The listing builds one solid part. Answer for the finished solid, in the listing's coordinates (mm). Face numbers are marked on the shaded views. A direction names the side the tool comes from. Round coordinates to 2 decimals unless told otherwise and drop trailing zeros. Write each loop counter-clockwise with the first axis right and the second up, starting at its lowest first coordinate (ties: lowest second). Pieces come first, ordered by that corner, then holes. Notation, with made-up numbers: (68, 7) - (126, 7) arc R32 cw to (126, 38) - close; hole circle Ø2 at (49, 79.5). An arc over 180 degrees is marked (long way). Return JSON: item names as keys, results as strings. Group by question number.
(1) Section B-B, the plane x = 28.5 is taken. Give the number of separate pieces and of enclosed holes in the cut face, then the cut area to 3 significant figures.
(2) Each of these flat-tipped pins is pushed along its axis until it touches: pin 1 (20 mm diameter, centred on y = -25.5, z = 6.5, fed in from +X); pin 2 (6 mm diameter, centred on x = -30.5, y = -12.5, fed in from +Z); pin 3 (3 mm diameter, centred on x = 7.5, y = -31.5, fed in from -Z). Where does it stop, or does it pass through?
(3) Determine the mould class of the marked faces 1, 2 and 3 for opening direction Z: +Z half, -Z half, draft (parallel to the pull), parting line (faces both ways), or undercut.
(4) Section A-A, the plane z = 0 is taken. Write down the section's boundary in (x, y), then the cut area to 3 significant figures.
(5) Which of the six approach directions +Z, -Z, +X, -X, +Y, -Y give full straight-line access (tool end or side, diameter ignored) to the marked faces 4, 5, 6 and 7?
(6) Find the intervals of material crossed by line 1 along Z through (x, y) = (0, -18) (3 decimals); line 2 along X through (y, z) = (-28.5, -25.5); line 3 along Z through (x, y) = (-0.5, -4), in increasing order. Write a range as [from, to].
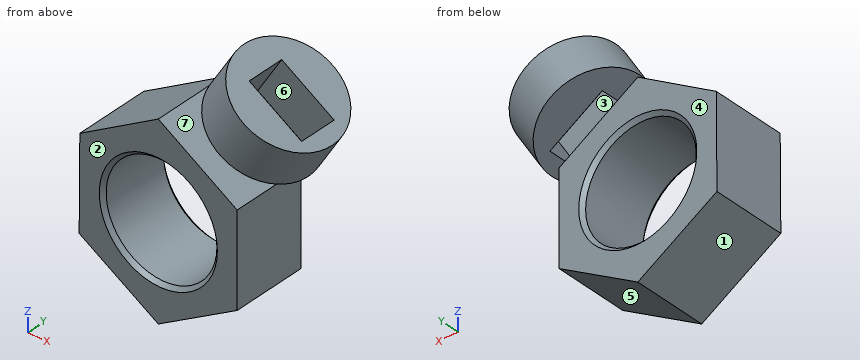
```python
from build123d import *

# Parameters (mm, degrees)
F0_R     = 30
F1_DEPTH = 40
F2_SIZE  = 2
F3_R     = 27.9010613337
F3_W     = 33.2406070083
F3_H     = 20.383390598
F4_DEPTH = 25


with BuildPart() as f1:
    # F0 (on Front) → F1 (new body)
    with BuildSketch(Plane.XZ):
        Polygon((0, 51.3005799085), (-42.5238697261, 25), (-42.8737902332, -24.9987755414), (0, -50.724990013), (42.7005271465, -24.7122050523), (42.7005271465, 25.2877949477), align=None)
        Circle(F0_R, mode=Mode.SUBTRACT)
    extrude(amount=F1_DEPTH)

    # F2
    f2_edges = [f1.edges().sort_by_distance(p)[0] for p in [
        (-30, -40, 0),
        (-30, 0, 0),
    ]]
    chamfer(f2_edges, length=F2_SIZE)

    # F3 (on face) → F4 (join)
    with BuildSketch(Plane(origin=(22.7930452708, 0, 37.4152575284), x_dir=(0.8540105429, 0, -0.5202556992), z_dir=(0.5202556992, 0, 0.8540105429))):
        Circle(F3_R)
        with Locations((2.8576394543, -0.7141805254)):
            Rectangle(F3_W, F3_H, mode=Mode.SUBTRACT)
    extrude(amount=F4_DEPTH)


solid = f1.part
```
Working result:
{
 "1": {"separate pieces": "3", "enclosed holes": "0", "area": "2,940 mm^2"},
 "2": {"pin 1": "stops at x = 42.7", "pin 2": "stops at z = 34.29", "pin 3": "stops at z = -47.07"},
 "3": {"face 1": "-Z half", "face 2": "draft", "face 3": "undercut"},
 "4": {"outline": "(-42.7, -40) - (-32, -40) - (-30, -38) - (-30, -2) - (-32, 0) - (-42.7, 0) - close; (30, -38) - (32, -40) - (42.7, -40) - (42.7, 0) - (32, 0) - (30, -2) - close", "area": "1,010 mm^2"},
 "5": {"face 4": "-Z, -X, +Y", "face 5": "-Z, +X, +Y, -Y", "face 6": "none", "face 7": "-Y"},
 "6": {"line 1": "z = [-50.725, -30], [30, 51.301]", "line 2": "x = [-42.04, -15.8], [15.8, 41.41]", "line 3": "z = [-50.42, -30], [30, 50.99], [51.61, 52.25]"}
}
